Work out the finished part from the listing and answer in its coordinate system (mm). Round coordinates to 2 decimals unless told otherwise and drop trailing zeros. Loops run counter-clockwise (first coordinate to the right, second up) from the corner with the lowest first, then second, coordinate; pieces in that order, holes last. Notation, with made-up numbers: (46.5, -19) - (90.5, -19) arc R30 cw to (90.5, 16) - close; hole circle Ø10 at (-24.5, -9.5). An arc over 180 degrees is marked (long way). Answer as CSV lines item,"result". Start each with the question number.
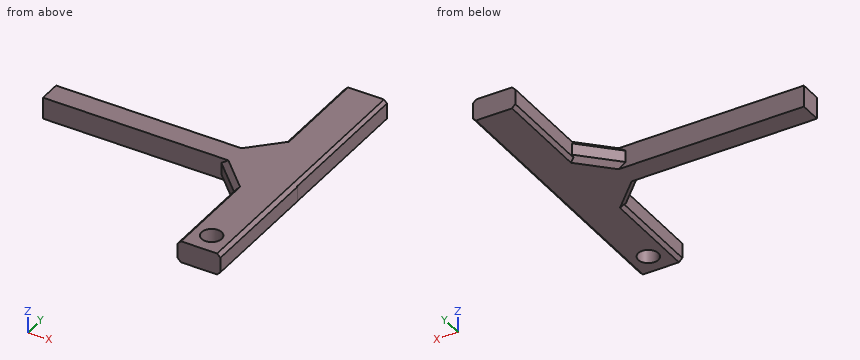
```python
from build123d import *

# Parameters (mm, degrees)
F0_R     = 3.020218
F1_DEPTH = 6.5
F2_SIZE  = 1.5
F3_SIZE  = 1


with BuildPart() as f1:
    # F0 (on Top) → F1 (new body)
    with BuildSketch(Plane.XY):
        Polygon((38.1, -3.25), (38.1, 3.25), (25.4, 3.25), (15.4, 3.25), (-38.1, 3.25), (-38.1, -3.25), (15.4, -3.25), (25.4, -3.25), align=None)
        Polygon((25.4, 3.25), (38.1, 3.25), (38.1, 41.35), (25.4, 41.35), (25.4, 13.25), align=None)
        Polygon((15.4, 3.25), (25.4, 3.25), (25.4, 13.25), align=None)
        Polygon((38.201772, -3.25), (38.1, -3.25), (25.4, -3.25), (25.4, -13.25), (25.4, -41.35), (38.201772, -41.35), align=None)
        with Locations((31.75, -35)):
            Circle(F0_R, mode=Mode.SUBTRACT)
        Polygon((25.4, -13.25), (25.4, -3.25), (15.4, -3.25), align=None)
    extrude(amount=F1_DEPTH)

    # F2
    f2_edges = [f1.edges().sort_by_distance(p)[0] for p in [
        (20.4, -8.25, 6.5),
        (20.4, 8.25, 6.5),
        (20.4, 8.25, 0),
        (20.4, -8.25, 0),
    ]]
    chamfer(f2_edges, length=F2_SIZE)

    # F3
    f3_edges = [f1.edges().sort_by_distance(p)[0] for p in [
        (25.4, -27.3, 6.5),
        (25.4, -27.3, 0),
        (25.4, 27.3, 6.5),
        (25.4, 27.3, 0),
        (38.201772, -22.3, 6.5),
        (38.201772, -22.3, 0),
    ]]
    chamfer(f3_edges, length=F3_SIZE)


solid = f1.part
```
Item 1: Section D-D, the plane x = -32.5 is taken. Give the vertices of the cut face in (y, z), and give its area (4 significant figures).
Item 2: Find the intervals of material crossed by L1, parallel to Y at x = 31.75, z = 4.5; L2, parallel to X at y = 18, z = 3.5; L3, parallel to X at y = -1.5, z = 3.5, in increasing order.
Item 3: Section B-B, the plane y = -35 is taken. Give the vertices of the cut face in (x, z), and give its area (3 significant figures).
Item 4: Flat-ended cylindrical pins translate along their axes: pin 1 Ø1 at (x, z) = (-4, 4.5) entering from -Y; pin 2 Ø2 at (x, z) = (11, 5.5) entering from -Y; pin 3 Ø1.4 at (y, z) = (27.5, 3) entering from +X; pin 4 Ø8 at (x, y) = (20, 16) entering from +Z. Find the tip coordinate at first contact, or state that the pin passes through.
Item 5: Section A-A, the plane x = 31.75 is taken. Give the vertices of the cut face in (y, z).
Item 6: Section C-C, the plane y = 22 is taken. Give the vertices of the cut face in (x, z), and give its area (3 significant figures).
Answer:
1,outline,"(-3.25, 0) - (3.25, 0) - (3.25, 6.5) - (-3.25, 6.5) - close"
1,area,"42.25 mm²"
2,L1,"y = -41.35 to -38.02, -31.98 to 41.35"
2,L2,"x = 25.4 to 38.1"
2,L3,"x = -38.1 to 38.1"
3,outline,"(25.4, 1) - (26.4, 0) - (28.73, 0) - (28.73, 6.5) - (26.4, 6.5) - (25.4, 5.5) - close; (34.77, 0) - (37.2, 0) - (38.2, 1) - (38.2, 5.5) - (37.2, 6.5) - (34.77, 6.5) - close"
3,area,"41.9 mm²"
4,pin 1,"stops at y = -3.25"
4,pin 2,"stops at y = -3.25"
4,pin 3,"stops at x = 38.1"
4,pin 4,"passes through"
5,outline,"(-41.35, 0) - (-38.02, 0) - (-38.02, 6.5) - (-41.35, 6.5) - close; (-31.98, 0) - (41.35, 0) - (41.35, 6.5) - (-31.98, 6.5) - close"
6,outline,"(25.4, 1) - (26.4, 0) - (37.2, 0) - (38.1, 0.9) - (38.1, 5.6) - (37.2, 6.5) - (26.4, 6.5) - (25.4, 5.5) - close"
6,area,"80.7 mm²"
